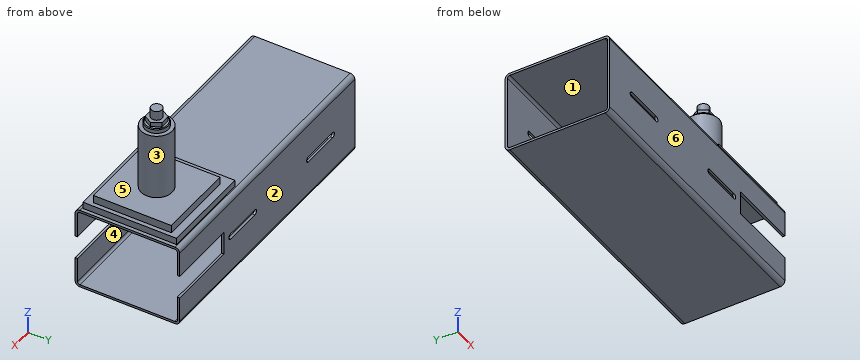
from build123d import *

# Parameters (mm, degrees)
F0_R           = 20
F1_DEPTH       = 85
F2_W           = 100
F2_H           = 100
F3_DEPTH       = 10
F4_W           = 120
F4_H           = 120
F5_DEPTH       = 10
F6_R           = 15
F7_DEPTH       = 6
F8_SIZE        = 1
F10_DEPTH      = 6
F11_R          = 7
F12_DEPTH      = 12
F14_DEPTH      = 60
F14_DEPTH_BACK = 300
F16_DEPTH      = 134.001
F17_W          = 182
F17_H          = 30
F18_DEPTH      = 134.001


with BuildPart() as f1:
    # F0 (on Top) → F1 (new body)
    with BuildSketch(Plane.XY):
        Circle(F0_R)
    extrude(amount=F1_DEPTH)

    # F2 (on Top) → F3 (join)
    with BuildSketch(Plane.XY):
        Rectangle(F2_W, F2_H)
    extrude(amount=-F3_DEPTH)

    # F4 (on face) → F5 (join)
    with BuildSketch(Plane(origin=(0, 0, -10), x_dir=(1, 0, 0), z_dir=(0, 0, -1))):
        with Locations((-4.663671, 0)):
            Rectangle(F4_W, F4_H)
    extrude(amount=F5_DEPTH)

    # F6 (on face) → F7 (join)
    with BuildSketch(Plane.XY.offset(85)):
        Circle(F6_R)
    extrude(amount=F7_DEPTH)

    # F8
    f8_edges = [f1.edges().sort_by_distance(p)[0] for p in [
        (-15, 0, 91),
    ]]
    chamfer(f8_edges, length=F8_SIZE)

    # F9 (on face) → F10 (join)
    with BuildSketch(Plane.XY.offset(91)):
        Polygon((-6.25, 10.825318), (-12.5, 0), (-6.25, -10.825318), (6.25, -10.825318), (12.5, 0), (6.25, 10.825318), align=None)
    extrude(amount=F10_DEPTH)

    # F11 (on face) → F12 (join)
    with BuildSketch(Plane.XY.offset(97)):
        Circle(F11_R)
    extrude(amount=F12_DEPTH)

    # F13 (on Right) → F14 (join, two sides)
    with BuildSketch(Plane.YZ) as f14_sk:
        with BuildLine():
            Line((61, -18.70025), (-61, -18.70025))
            ThreePointArc((-61, -18.70025), (-65.242641, -20.457609), (-67, -24.70025))
            Line((-67, -24.70025), (-67, -118.70025))
            ThreePointArc((-67, -118.70025), (-65.242641, -122.94289), (-61, -124.70025))
            Line((-61, -124.70025), (61, -124.70025))
            ThreePointArc((61, -124.70025), (65.242641, -122.94289), (67, -118.70025))
            Line((67, -118.70025), (67, -24.70025))
            ThreePointArc((67, -24.70025), (65.242641, -20.457609), (61, -18.70025))
        make_face()
        with BuildLine():
            Line((-64, -118.70025), (-64, -24.70025))
            ThreePointArc((-64, -24.70025), (-63.12132, -22.578929), (-61, -21.70025))
            Line((-61, -21.70025), (61, -21.70025))
            ThreePointArc((61, -21.70025), (63.12132, -22.578929), (64, -24.70025))
            Line((64, -24.70025), (64, -118.70025))
            ThreePointArc((64, -118.70025), (63.12132, -120.82157), (61, -121.70025))
            Line((61, -121.70025), (-61, -121.70025))
            ThreePointArc((-61, -121.70025), (-63.12132, -120.82157), (-64, -118.70025))
        make_face(mode=Mode.SUBTRACT)
    extrude(amount=F14_DEPTH)
    extrude(f14_sk.sketch, amount=-F14_DEPTH_BACK)

    # F15 (on face) → F16 (cut, through all)
    with BuildSketch(Plane.XZ.offset(67)):
        with BuildLine():
            ThreePointArc((-254.5, -68.2), (-258, -71.7), (-254.5, -75.2))
            Line((-254.5, -75.2), (-204.5, -75.2))
            ThreePointArc((-204.5, -75.2), (-201, -71.7), (-204.5, -68.2))
            Line((-204.5, -68.2), (-254.5, -68.2))
        make_face()
        with BuildLine():
            Line((-44.500257, -67.913005), (-94.500257, -67.913005))
            ThreePointArc((-94.500257, -67.913005), (-98.000257, -71.413005), (-94.500257, -74.913005))
            Line((-94.500257, -74.913005), (-44.500257, -74.913005))
            ThreePointArc((-44.500257, -74.913005), (-41.000257, -71.413005), (-44.500257, -67.913005))
        make_face()
    extrude(amount=-F16_DEPTH, mode=Mode.SUBTRACT)

    # F17 (on face) → F18 (cut, through all)
    with BuildSketch(Plane.XZ.offset(67)):
        with Locations((60, -71.70025)):
            Rectangle(F17_W, F17_H)
    extrude(amount=-F18_DEPTH, mode=Mode.SUBTRACT)


solid = f1.part
The listing builds one solid part. Answer for the finished solid, in the listing's coordinates (mm). Face numbers are marked on the shaded views. A direction names the side the tool comes from. Coordinates: 2 decimals unless noted, no trailing zeros. Loops run counter-clockwise (first coordinate to the right, second up) from the corner with the lowest first, then second, coordinate; pieces in that order, holes last.
1) A tool of negligible diameter and unlimited length cuts with its end or side. For the marked faces 1, 2 and 3, from which of +Z, -Z, +X, -X, +Y, -Y can it reach the whole face along a straight path? Write none if from no direction.
2) Find the intervals of material crossed by L1, parallel to Z at x = 34, y = 39; L2, parallel to Z at x = -204, y = -39; L3, parallel to Y at x = -207, z = -110, in increasing order.
3) Flat-ended cylindrical pins translate along their axes: pin 1 Ø8 at (x, z) = (7.5, -9.5) entering from +Y; pin 2 Ø3.5 at (x, y) = (13.5, 65) entering from +Z; pin 3 Ø1.5 at (x, y) = (7, -66) entering from -Z. Find the tip coordinate at first contact, or state that the pin passes through.
4) Find section B-B on y = -36. Write down the section's boundary in (x, z), then the cut area to 3 significant figures.
5) Find section D-D on z = -80.5. Write down the section's boundary in (x, y), then the cut area to 3 significant figures.
6) Find section C-C on x = -87. Write down the section's boundary in (y, z), then the cut area to 3 significant figures.
7) Determine the mould class of the marked faces 4, 5 and 6 for opening direction Z: pulls with the +Z half, pulls with the -Z half, needs draft (parallel to the pull), parting line crosses it, or undercut.
8) Find section A-A on x = -141.5. Write down the section's boundary in (y, z).
Values:
1. face 1: +X, -X
1. face 2: +Z, -Z, +X, -X, +Y
1. face 3: +Z
2. L1: z = -124.7 to -121.7, -21.7 to 0
2. L2: z = -124.7 to -121.7, -21.7 to -18.7
2. L3: y = -67 to -64, 64 to 67
3. pin 1: stops at y = 60
3. pin 2: stops at z = -19.14
3. pin 3: stops at z = -122.94
4. outline: (-300, -124.7) - (60, -124.7) - (60, -121.7) - (-300, -121.7) - close; (-300, -21.7) - (60, -21.7) - (60, -18.7) - (55.34, -18.7) - (55.34, -10) - (50, -10) - (50, 0) - (-50, 0) - (-50, -10) - (-64.66, -10) - (-64.66, -18.7) - (-300, -18.7) - close
4. area: 4,200 mm2
5. outline: (-300, -67) - (-31, -67) - (-31, -64) - (-300, -64) - close; (-300, 64) - (-31, 64) - (-31, 67) - (-300, 67) - close
5. area: 1,610 mm2
6. outline: (-67, -118.7) arc R6 ccw to (-61, -124.7) - (61, -124.7) arc R6 ccw to (67, -118.7) - (67, -74.91) - (64, -74.91) - (64, -118.7) arc R3 cw to (61, -121.7) - (-61, -121.7) arc R3 cw to (-64, -118.7) - (-64, -74.91) - (-67, -74.91) - close; (-67, -67.91) - (-64, -67.91) - (-64, -24.7) arc R3 cw to (-61, -21.7) - (61, -21.7) arc R3 cw to (64, -24.7) - (64, -67.91) - (67, -67.91) - (67, -24.7) arc R6 ccw to (61, -18.7) - (-61, -18.7) arc R6 ccw to (-67, -24.7) - close
6. area: 1,340 mm2
7. face 4: undercut
7. face 5: pulls with the +Z half
7. face 6: needs draft
8. outline: (-67, -118.7) arc R6 ccw to (-61, -124.7) - (61, -124.7) arc R6 ccw to (67, -118.7) - (67, -24.7) arc R6 ccw to (61, -18.7) - (-61, -18.7) arc R6 ccw to (-67, -24.7) - close; hole (-64, -118.7) arc R3 ccw to (-61, -121.7) - (61, -121.7) arc R3 ccw to (64, -118.7) - (64, -24.7) arc R3 ccw to (61, -21.7) - (-61, -21.7) arc R3 ccw to (-64, -24.7) - close
